Geometry: final body of the model. Coordinates: model frame, mm. Coordinates: 2 decimals unless noted, no trailing zeros. Loops run counter-clockwise (first coordinate to the right, second up) from the corner with the lowest first, then second, coordinate; pieces in that order, holes last. Notation, with made-up numbers: (34, 25) -> (58, 25) arc R32 ccw to (58, 54) -> close; hole circle Ø3 at (13.5, 52). An arc over 180 degrees is marked (long way). One line per item, written item: value. Start each with the question number.
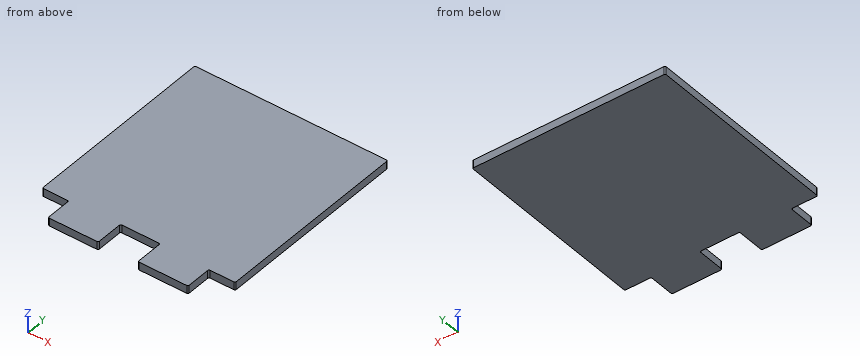
Autodesk Inventor part; units mm, degrees
sketch "Sketch1" plane through (0, 0, 0) normal (0, 0, 1) x (1, 0, 0)
  line L0 (-73, 83.75) -> (73, 83.75)
  line L1 (73, 83.75) -> (73, -83.75)
  line L2 (73, -83.75) -> (-73, -83.75)
  line L3 (-73, -83.75) -> (-73, 83.75)
  point P0 (0, 83.75)
  point P1 (0, 0)
  point P2 (-73, 0)
  dimension "d0" = 146
  dimension "d1" = 167.5
extrude "Extrusion1" add sketch "Sketch1" along normal blind 6
sketch "Sketch2" plane through (0, 0, 6) normal (0, 0, 1) x (1, 0, 0)
  line L0 (-73, 83.75) -> (-73, -83.75)
  line L1 (-73, -83.75) -> (-73, -63.75)
  line L2 (-67.5, -78.25) -> (-53, -78.25)
  line L3 (-53, -78.25) -> (-53, -83.75)
  line L4 (-73, -63.75) -> (-53, -63.75)
  line L5 (-53, -63.75) -> (-53, -83.75)
  line L6 (-73, -83.75) -> (73, -83.75)
  line L7 (-53, -83.75) -> (-73, -83.75)
  point P0 (0, 0)
  point P1 (40.5, -62.5)
  dimension "d14" = 20
  dimension "d18" = 20
extrude "Extrusion2" cut sketch "Sketch2" against normal blind 6
mirror "Mirror1" about plane through (0, 0, 0) normal (1, 0, 0) of "Extrusion2"
sketch "Sketch4" plane through (0, 0, 0) normal (0, 0, -1) x (-1, 0, 0)
  line L0 (-15, -62.25) -> (15, -62.25)
  line L1 (15, -62.25) -> (15, -83.75)
  line L2 (15, -83.75) -> (-15, -83.75)
  line L3 (-15, -83.75) -> (-15, -62.25)
  line L4 (53, -83.75) -> (-53, -83.75)
  point P0 (0, 0)
  point P1 (0, -83.75)
  point P2 (0, -83.75)
  point P3 (0, -83.75)
  dimension "d19" = 30
  dimension "d20" = 21.5
extrude "Extrusion4" cut sketch "Sketch4" against normal blind 6
fillet "Fillet1" radius 1 12 edges at (73, -63.75, 3) (53, -63.75, 3) (53, -83.75, 3) (15, -83.75, 3) (-15, -83.75, 3) (-15, -62.25, 3) (-53, -83.75, 3) (15, -62.25, 3) (-53, -63.75, 3) (-73, -63.75, 3) (-73, 83.75, 3) (73, 83.75, 3)
properties part number "MDF_Front_Side" material "MDF Medium Density Fiberboard"
1. Line query: L1, parallel to X at y = -72, z = 2.7; L2, parallel to Y at x = 61, z = 4.8; L3, parallel to Y at x = 6, z = 4.1. Output: solid intervals per line, ascending. Write a range as [from, to].
2. Section C-C on x = -57.5. Return the cut outline in (y, z), plus the area to 3 significant figures.
3. Pin query (flat end, axial travel): pin 1 Ø3 at (y, z) = (-76, 4) entering from +X; pin 2 Ø1.8 at (x, z) = (65, 3) entering from -Y; pin 3 Ø3 at (x, z) = (3.5, 4) entering from -Y. Return the tip coordinate at first contact, or that it passes through.
4. Section A-A on y = -68.5. Return the cut outline in (x, z), plus the area to 3 significant figures.
5. Section B-B on z = 4.5. Return the cut outline in (x, y), plus the area to 3 significant figures.
6. Section D-D on x = -9. Return the cut outline in (y, z), plus the area to 3 significant figures.
Checks:
1. L1: [-53, -15], [15, 53]
1. L2: [-63.75, 83.75]
1. L3: [-62.25, 83.75]
2. outline: (-63.75, 0) -> (83.75, 0) -> (83.75, 6) -> (-63.75, 6) -> close
2. area: 885 mm²
3. pin 1: x = 53
3. pin 2: y = -63.75
3. pin 3: y = -62.25
4. outline: (-53, 0) -> (-15, 0) -> (-15, 6) -> (-53, 6) -> close; (15, 0) -> (53, 0) -> (53, 6) -> (15, 6) -> close
4. area: 456 mm²
5. outline: (-73, -62.75) arc R1 ccw to (-72, -63.75) -> (-54, -63.75) arc R1 cw to (-53, -64.75) -> (-53, -82.75) arc R1 ccw to (-52, -83.75) -> (-16, -83.75) arc R1 ccw to (-15, -82.75) -> (-15, -63.25) arc R1 cw to (-14, -62.25) -> (14, -62.25) arc R1 cw to (15, -63.25) -> (15, -82.75) arc R1 ccw to (16, -83.75) -> (52, -83.75) arc R1 ccw to (53, -82.75) -> (53, -64.75) arc R1 cw to (54, -63.75) -> (72, -63.75) arc R1 ccw to (73, -62.75) -> (73, 82.75) arc R1 ccw to (72, 83.75) -> (-72, 83.75) arc R1 ccw to (-73, 82.75) -> close
5. area: 23,000 mm²
6. outline: (-62.25, 0) -> (83.75, 0) -> (83.75, 6) -> (-62.25, 6) -> close
6. area: 876 mm²
